```python
from build123d import *

# Parameters (mm, degrees)
SKETCH1_R      = 25
EXTRUDE1_DEPTH = 110
SKETCH2_R      = 20
EXTRUDE2_DEPTH = 5
EXTRUDE3_DEPTH = 90
EXTRUDE4_DEPTH = 91


with BuildPart() as part:
    # Sketch1 → Extrude1 (new body)
    with BuildSketch(Plane.XY):
        Circle(SKETCH1_R)
    extrude(amount=EXTRUDE1_DEPTH)

    # Sketch2 → Extrude2 (cut)
    with BuildSketch(Plane.XY.offset(110)):
        Circle(SKETCH2_R)
    extrude(amount=-EXTRUDE2_DEPTH, mode=Mode.SUBTRACT)

    # Sketch3 → Extrude3 (add)
    with BuildSketch(Plane.XY):
        with BuildLine():
            Line((-20, -100), (-20, 0))
            Line((-20, 0), (20, 0))
            Line((20, 0), (20, -100))
            ThreePointArc((20, -100), (0, -120), (-20, -100))
        make_face()
    extrude(amount=EXTRUDE3_DEPTH)

    # Sketch4 → Extrude4 (cut, through all)
    with BuildSketch(Plane.XY.offset(90)):
        with BuildLine():
            Line((-15, -20), (-15, -100))
            ThreePointArc((-15, -100), (0, -115), (15, -100))
            Line((15, -100), (15, -20))
            ThreePointArc((15, -20), (0, -25), (-15, -20))
        make_face()
    extrude(amount=-EXTRUDE4_DEPTH, mode=Mode.SUBTRACT)


solid = part.part
```
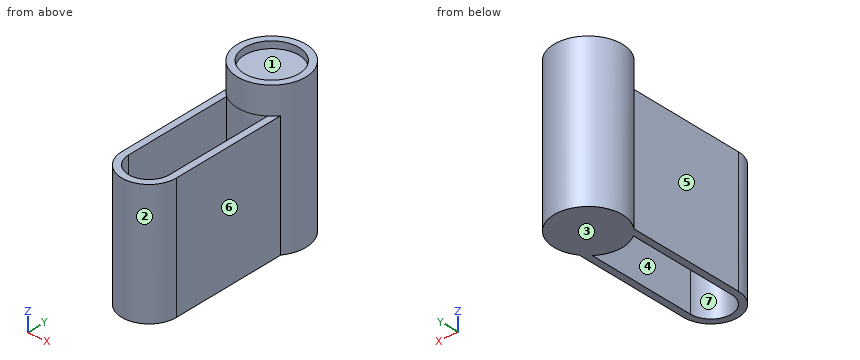
Model file for the job. Use its own axes, mm. Face numbers are marked on the shaded views. A direction names the side the tool comes from. Coordinates: 2 decimals unless noted, no trailing zeros. Write each loop counter-clockwise with the first axis right and the second up, starting at its lowest first coordinate (ties: lowest second). Pieces come first, ordered by that corner, then holes. Notation, with made-up numbers: (10.5, -29) - (30.5, -29) arc R22 ccw to (30.5, -1) - close; hole circle Ø5 at (41.25, 19). An arc over 180 degrees is marked (long way). One line per item, written item: value. Start each with the question number.
1. Slice it at A-A (y = -84.5). Write the cut outline in (x, z), plus the area to 3 significant figures.
2. Tool access for the marked faces 5, 6 and 7: list every direction of +Z, -Z, +X, -X, +Y, -Y with a clear straight run to the whole face (end or side of a thin tool).
3. Flat gauge pins, fed straight in: pin 1 (5 mm diameter, centred on y = 9, z = 32, fed in from -X); pin 2 (1 mm diameter, centred on x = 6.5, z = 66, fed in from -Y); pin 3 (1.5 mm diameter, centred on y = -52.5, z = 15.5, fed in from -X). Where does each tip first touch, or does it go through?
4. Slice it at D-D (y = 0). Write the cut outline in (x, z).
5. Slice it at C-C (z = 13.5). Write the cut outline in (x, y).
6. Mould opens along Y. For the marked faces 1, 2, 3 and 4 say: released by +Y, released by -Y, zero draft, split by the parting line, or undercut.
7. Slice it at B-B (x = 0). Write the cut outline in (y, z).
8. Probe line 1 (Y direction, x = 0, z = 109); line 2 (Z direction, x = -2, y = 18); line 3 (X direction, y = -28.5, z = 53). List the from-to ranges inside material, lowest first. Write a range as from..to.
Answers below:
1. outline: (-20, 0) - (-15, 0) - (-15, 90) - (-20, 90) - close; (15, 0) - (20, 0) - (20, 90) - (15, 90) - close
1. area: 900 mm^2
2. face 5: +Z, -Z, -X, -Y
2. face 6: +Z, -Z, +X, -Y
2. face 7: +Z, -Z
3. pin 1: stops at x = -24.14
3. pin 2: stops at y = -119.08
3. pin 3: stops at x = -20
4. outline: (-25, 0) - (25, 0) - (25, 110) - (20, 110) - (20, 105) - (-20, 105) - (-20, 110) - (-25, 110) - close
5. outline: (-20, -100) arc R20 ccw to (20, -100) - (20, -15) arc R25 ccw (long way) to (-20, -15) - close; hole (-15, -100) arc R15 ccw to (15, -100) - (15, -20) arc R25 cw to (-15, -20) - close
6. face 1: undercut
6. face 2: released by -Y
6. face 3: zero draft
6. face 4: undercut
7. outline: (-120, 0) - (-115, 0) - (-115, 90) - (-120, 90) - close; (-25, 0) - (25, 0) - (25, 110) - (20, 110) - (20, 105) - (-20, 105) - (-20, 110) - (-25, 110) - close
8. line 1: y = -25..-20, 20..25
8. line 2: z = 0..105
8. line 3: x = -20..-15, 15..20
